Check sheet for the modelled part. Datum: model origin and axes. Units: mm. Face numbers are marked on the shaded views. Coordinates: 2 decimals unless noted, no trailing zeros. Loops run counter-clockwise (first coordinate to the right, second up) from the corner with the lowest first, then second, coordinate; pieces in that order, holes last.
```python
from build123d import *

# Parameters (mm, degrees)
ESQUISSE1_R                    = 23
ESQUISSE1_R_2                  = 20
BOSS_EXTRU_1_DEPTH             = 25
BOSS_EXTRU_2_REACH             = 48
ESQUISSE2_R                    = 5
BOSS_EXTRU_2_DIRECTION_2_DEPTH = 5


with BuildPart() as part:
    # Esquisse1 → Boss.-Extru.1 (new body, symmetric)
    with BuildSketch(Plane.XY):
        Circle(ESQUISSE1_R)
        Circle(ESQUISSE1_R_2, mode=Mode.SUBTRACT)
    extrude(amount=BOSS_EXTRU_1_DEPTH, both=True)

    # Esquisse2 → Boss.-Extru.2 (add, up to next)
    with BuildSketch(Plane(origin=(23, 0, 0), x_dir=(0, 0, -1), z_dir=(1, 0, 0)), mode=Mode.PRIVATE) as boss_extru_2_sk1:
        Circle(ESQUISSE2_R)
    boss_extru_2_tool1 = extrude(boss_extru_2_sk1.sketch, amount=-BOSS_EXTRU_2_REACH, mode=Mode.PRIVATE) - part.part
    add(boss_extru_2_tool1.solids().sort_by_distance((23, 0, 0))[0])
    add(boss_extru_2_tool1.solids().sort_by_distance((23, 0, 0))[1])

    # Esquisse2 → Boss.-Extru.2 direction 2 (add)
    with BuildSketch(Plane(origin=(23, 0, 0), x_dir=(0, 0, -1), z_dir=(1, 0, 0))):
        Circle(ESQUISSE2_R)
    extrude(amount=BOSS_EXTRU_2_DIRECTION_2_DEPTH)


solid = part.part
```
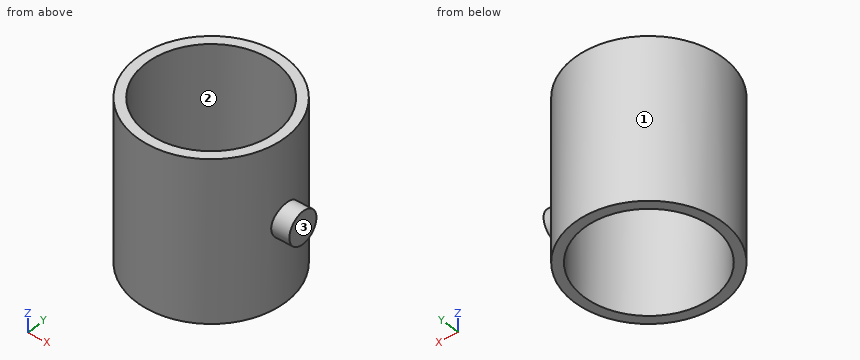
1) Section check C-C on z = 0. Enter the section's corners in (x, y), plus the area to 3 significant figures.
Answer sheet:
outline: (22.45, -5) - (28, -5) - (28, 5) - (22.45, 5) arc R23 ccw (long way) to start; hole circle Ø40 at (0, 0)
area: 457 mm2
2) Scan lines: line 1 (Y direction, x = 0, z = 13); line 2 (Y direction, x = 4, z = 17); line 3 (X direction, y = 7, z = 21.5) (3 decimals). Record each from-to range of solid material in increasing order.
Answer sheet:
line 1: y = -23 to -20, 20 to 23
line 2: y = -22.65 to -19.6, 19.6 to 22.65
line 3: x = -21.909 to -18.735, 18.735 to 21.909
3) Section check D-D on y = -4. Enter the section's corners in (x, z).
Answer sheet:
outline: (-22.65, -25) - (-19.6, -25) - (-19.6, 25) - (-22.65, 25) - close; (19.6, -25) - (22.65, -25) - (22.65, -3) - (28, -3) - (28, 3) - (22.65, 3) - (22.65, 25) - (19.6, 25) - close
4) Depth check by flat-ended pin: pin 1 (1.5 mm diameter, centred on x = 14, z = 8.5, fed in from -Y); pin 2 (4 mm diameter, centred on y = 18, z = -6, fed in from +X); pin 3 (24 mm diameter, centred on x = 0, y = 0, fed in from +Z); pin 4 (12 mm diameter, centred on x = 13, z = -4.5, fed in from -Y). Enter the tip coordinate at first touch or a pass-through.
Answer sheet:
pin 1: stops at y = -18.8
pin 2: stops at x = 16.52
pin 3: passes through
pin 4: stops at y = -21.91
5) Section check A-A on x = 0. Enter the section's corners in (y, z), plus the area to 3 significant figures.
Answer sheet:
outline: (-23, -25) - (-20, -25) - (-20, 25) - (-23, 25) - close; (20, -25) - (23, -25) - (23, 25) - (20, 25) - close
area: 300 mm2
6) Section check B-B on y = 17. Enter the section's corners in (x, z).
Answer sheet:
outline: (-15.49, -25) - (-10.54, -25) - (-10.54, 25) - (-15.49, 25) - close; (10.54, -25) - (15.49, -25) - (15.49, 25) - (10.54, 25) - close
7) Mould release check, pull along X, two halves, no side actions. Record for the marked faces 1, 2 and 3: +X half, -X half, draft (parallel to the pull), parting line (faces both ways), or undercut.
Answer sheet:
face 1: parting line
face 2: undercut
face 3: +X half
